```python
from build123d import *

# Parameters (mm, degrees)
SKETCH1_R           = 18.5
BOSS_EXTRUDE1_DEPTH = 8
SKETCH11_R          = 1.67
CUT_EXTRUDE5_DEPTH  = 1.15
CIRPATTERN1_COUNT   = 4
SKETCH13_W          = 22
SKETCH13_H          = 22
SKETCH13_W_2        = 20.9
SKETCH13_H_2        = 20.9
BOSS_EXTRUDE3_DEPTH = 1.3
SKETCH12_W          = 22
SKETCH12_H          = 22
BOSS_EXTRUDE2_DEPTH = 0.8
CUT_EXTRUDE6_DEPTH  = 28.603260677


with BuildPart() as part:
    # Sketch1 → Boss-Extrude1 (new body)
    with BuildSketch(Plane(origin=(0, 0, 0), x_dir=(1, 0, 0), z_dir=(0, 1, 0))):
        with Locations(Location((0, 0, 0), (0, 0, 270))):
            Circle(SKETCH1_R)
    extrude(amount=BOSS_EXTRUDE1_DEPTH)

    # Sketch11 → Cut-Extrude5 (cut)
    with BuildSketch(Plane(origin=(0, 8, 0), x_dir=(1, 0, 0), z_dir=(0, 1, 0))):
        with Locations(Location((0.066774753, 15.781335524, 0), (0, 0, 270))):
            Circle(SKETCH11_R)
    cut_extrude5 = extrude(amount=-CUT_EXTRUDE5_DEPTH, mode=Mode.SUBTRACT)

    # CirPattern1: Cut-Extrude5 ×4 about axis
    cirpattern1_axis = Axis((0, 0, 0), (0, 1, 0))
    for i in range(1, CIRPATTERN1_COUNT):
        add(cut_extrude5.rotate(cirpattern1_axis, i * 360 / CIRPATTERN1_COUNT), mode=Mode.SUBTRACT)

    # Sketch13 → Boss-Extrude3 (add)
    with BuildSketch(Plane(origin=(0, 8, 0), x_dir=(1, 0, 0), z_dir=(0, 1, 0))):
        Rectangle(SKETCH13_W, SKETCH13_H)
        Rectangle(SKETCH13_W_2, SKETCH13_H_2, mode=Mode.SUBTRACT)
    extrude(amount=BOSS_EXTRUDE3_DEPTH)

    # Sketch12 → Boss-Extrude2 (add)
    with BuildSketch(Plane(origin=(0, 8, 0), x_dir=(1, 0, 0), z_dir=(0, 1, 0))):
        Rectangle(SKETCH12_W, SKETCH12_H)
    extrude(amount=BOSS_EXTRUDE2_DEPTH)

    # Sketch14 → Cut-Extrude6 (cut, through all)
    with BuildSketch(Plane(origin=(0, 8.8, 0), x_dir=(1, 0, 0), z_dir=(0, 1, 0))):
        with BuildLine():
            ThreePointArc((-9, -7.85), (-8.663172798, -8.663172798), (-7.85, -9))
            Line((-7.85, -9), (7.85, -9))
            ThreePointArc((7.85, -9), (8.663172798, -8.663172798), (9, -7.85))
            Line((9, -7.85), (9, 7.85))
            ThreePointArc((9, 7.85), (8.663172798, 8.663172798), (7.85, 9))
            Line((7.85, 9), (-7.85, 9))
            ThreePointArc((-7.85, 9), (-8.663172798, 8.663172798), (-9, 7.85))
            Line((-9, 7.85), (-9, -7.85))
        make_face()
    extrude(amount=-CUT_EXTRUDE6_DEPTH, mode=Mode.SUBTRACT)


solid = part.part
```
The listing builds one solid part. Answer for the finished solid, in the listing's coordinates (mm). A direction names the side the tool comes from. Coordinates: 2 decimals unless noted, no trailing zeros. Loops run counter-clockwise (first coordinate to the right, second up) from the corner with the lowest first, then second, coordinate; pieces in that order, holes last. Notation, with made-up numbers: (-8.75, 74.25) -> (30.25, 74.25) arc R15 ccw to (30.25, 100.25) -> close; hole circle Ø7 at (64.5, 61). An arc over 180 degrees is marked (long way). Use one line per item in the form item = value. Start each with the question number.
Item 1: The part is cut by section C-C on y = 7.5. Determine the outline of the cut face in (x, z).
Item 2: Flat-ended cylindrical pins translate along their axes: pin 1 Ø1 at (y, z) = (4.5, 8.5) entering from +X; pin 2 Ø2.5 at (y, z) = (6, 3.5) entering from +X; pin 3 Ø1.5 at (y, z) = (1, 4.5) entering from +X. Find the tip coordinate at first contact, or state that the pin passes through.
Item 3: The part is cut by section A-A on z = -8.5. Determine the outline of the cut face in (x, y).
Item 4: A tool of negligible diameter and unlimited length cuts with its end or side. For faces 5 (the face through (0, 9, -11)), 6 (the face through (-17.45, 7.43, -0.14)), 7 (the face through (-9, 4, 0)), from which of +Z, -Z, +X, -X, +Y, -Y can it reach the whole face along a straight path? Write none if from no direction.
Item 5: The mould has two halves that part along X. Classify faces 1 (the face through (0.14, 7.43, -17.45)), 2 (the face through (-11, 9, 0)), 3 (the face through (0, 9, 11)), 4 (the face through (8.672, 4.462, -8.654)): released by +X, released by -X, zero draft, split by the parting line, or undercut.
Item 6: The part is cut by section D-D on z = 16. Determine the outline of the cut face in (x, y), then the cut area to 3 significant figures.
Item 7: The part is cut by section B-B on y = 1.75. Determine the outline of the cut face in (x, z), then the cut area to 3 significant figures.
Item 8: Consider L1, parallel to Z at x = 4, y = 1.25; L2, parallel to Z at x = -3.5, y = 4.75; L3, parallel to X at y = 1.75, z = -8.5. Determine where each line is inside the solid, lowest interval first. Write a range as [from, to].
Answer key:
q1.outline = circle Ø37 at (0, 0); hole circle Ø3.34 at (-15.78, -0.07); hole (-9, -7.85) arc R1.15 ccw to (-7.85, -9) -> (7.85, -9) arc R1.15 ccw to (9, -7.85) -> (9, 7.85) arc R1.15 ccw to (7.85, 9) -> (-7.85, 9) arc R1.15 ccw to (-9, 7.85) -> close; hole circle Ø3.34 at (-0.07, 15.78); hole circle Ø3.34 at (0.07, -15.78); hole circle Ø3.34 at (15.78, 0.07)
q2.pin_1 = 16.68
q2.pin_2 = 18.36
q2.pin_3 = 18.12
q3.outline = (-16.43, 0) -> (-8.8, 0) -> (-8.8, 8.8) -> (-10.45, 8.8) -> (-10.45, 9.3) -> (-11, 9.3) -> (-11, 8) -> (-16.43, 8) -> close; (8.8, 0) -> (16.43, 0) -> (16.43, 8) -> (11, 8) -> (11, 9.3) -> (10.45, 9.3) -> (10.45, 8.8) -> (8.8, 8.8) -> close
q4.face_5 = -Z, +X, -X, +Y
q4.face_6 = +Y
q4.face_7 = +Y, -Y
q5.face_1 = undercut
q5.face_2 = released by -X
q5.face_3 = zero draft
q5.face_4 = undercut
q6.outline = (-9.29, 0) -> (9.29, 0) -> (9.29, 8) -> (1.59, 8) -> (1.59, 6.85) -> (-1.72, 6.85) -> (-1.72, 8) -> (-9.29, 8) -> close
q6.area = 145 mm2
q7.outline = circle Ø37 at (0, 0); hole (-9, -7.85) arc R1.15 ccw to (-7.85, -9) -> (7.85, -9) arc R1.15 ccw to (9, -7.85) -> (9, 7.85) arc R1.15 ccw to (7.85, 9) -> (-7.85, 9) arc R1.15 ccw to (-9, 7.85) -> close
q7.area = 752 mm2
q8.L1 = [-18.06, -9], [9, 18.06]
q8.L2 = [-18.17, -9], [9, 18.17]
q8.L3 = [-16.43, -8.8], [8.8, 16.43]
